```python
from build123d import *

# Parameters (mm, degrees)
SKETCH2_W           = 100
SKETCH2_H           = 200
BOSS_EXTRUDE1_DEPTH = 75
SKETCH5_R           = 2.5
SKETCH3_R           = 10
SKETCH6_R           = 2.5
CUT_EXTRUDE1_DEPTH  = 4


with BuildPart() as part:
    # Sketch2 → Boss-Extrude1 (new body)
    with BuildSketch(Plane(origin=(0, 0, 0), x_dir=(1, 0, 0), z_dir=(0, 1, 0))):
        Rectangle(SKETCH2_W, SKETCH2_H)
    extrude(amount=BOSS_EXTRUDE1_DEPTH)

    # Sketch5 → Loft1 section 0
    with BuildSketch(Plane.ZY.offset(55)):
        with Locations((0, 15)):
            Circle(SKETCH5_R)
    # Sketch3 → Loft1 section 1
    with BuildSketch(Plane.ZY.offset(50)):
        with Locations((0, 15)):
            Circle(SKETCH3_R)
    loft1 = loft()

    # Sketch6 → Cut-Extrude1 (cut)
    with BuildSketch(Plane.ZY.offset(55)):
        with Locations((0, 15)):
            Circle(SKETCH6_R)
    cut_extrude1 = extrude(amount=-CUT_EXTRUDE1_DEPTH, mode=Mode.SUBTRACT)

    # Mirror1: Loft1, Cut-Extrude1 across plane
    add(loft1.mirror(Plane(origin=(0, 0, 0), x_dir=(0, 0, 1), z_dir=(1, 0, 0))))
    add(cut_extrude1.mirror(Plane(origin=(0, 0, 0), x_dir=(0, 0, 1), z_dir=(1, 0, 0))), mode=Mode.SUBTRACT)


solid = part.part
```
Geometry check sheet. Reference: the model listing, model coordinates, mm. A direction names the side the tool comes from. Coordinates: 2 decimals unless noted, no trailing zeros. Write each loop counter-clockwise with the first axis right and the second up, starting at its lowest first coordinate (ties: lowest second). Pieces come first, ordered by that corner, then holes. Notation, with made-up numbers: M 9,48 L 26,48 A25 ccw 26,80 Z; hole C -18.75,32.25 d8. An arc over 180 degrees is marked long. Answer as a JSON object with one key per item and string values.
1. Section check B-B, the plane y = 56. Enter the section's corners in (x, z), plus the area to 3 significant figures.
Answers below:
{"outline": "M -50,-100 L 50,-100 L 50,100 L -50,100 Z", "area": "20,000 mm²"}
2. Tool access check on faces 5 (the cylindrical face through (53.03, 12.56, -0.54)), 6 (the flat face through (-1, 37, 100)), 7 (the flat face through (-51, 15, 0)). Record the directions out of +Z, -Z, +X, -X, +Y, -Y that give a thin tool (end or side, any length) a straight path to the whole face; none if there is none.
Answers below:
{"face 5": "+X", "face 6": "+Z, +X, -X, +Y, -Y", "face 7": "-X"}
3. Section check C-C, the plane z = 82.5. Enter the section's corners in (x, y), plus the area to 3 significant figures.
Answers below:
{"outline": "M -50,0 L 50,0 L 50,75 L -50,75 Z", "area": "7,500 mm²"}
4. Go/stop test with flat-tipped pins: pin 1 Ø4.5 at (y, z) = (15, 0) entering from +X; pin 2 Ø1.5 at (y, z) = (14.5, 1) entering from -X; pin 3 Ø5 at (y, z) = (8, 67) entering from +X. Record where each tip stops, or that it passes through.
Answers below:
{"pin 1": "stops at x = 51", "pin 2": "stops at x = -51", "pin 3": "stops at x = 50"}
5. Section check A-A, the plane z = 0. Enter the section's corners in (x, y), plus the area to 4 significant figures.
Answers below:
{"outline": "M -55,12.5 L -50,5 L -50,0 L 50,0 L 50,5 L 55,12.5 L 51,12.5 L 51,17.5 L 55,17.5 L 50,25 L 50,75 L -50,75 L -50,25 L -55,17.5 L -51,17.5 L -51,12.5 Z", "area": "7,585 mm²"}
6. Scan lines: L1, parallel to X at y = 23, z = 67.5; L2, parallel to Y at x = -53.45, z = 0 (3 decimals); L3, parallel to Y at x = -54, z = 0. Record each from-to range of solid material in increasing order.
Answers below:
{"L1": "x = -50 to 50", "L2": "y = 10.175 to 12.5, 17.5 to 19.825", "L3": "y = 11 to 12.5, 17.5 to 19"}
7. Draft check along Z on faces 1 (the flat face through (51, 15, 0)), 2 (the cylindrical face through (-53.03, 12.56, -0.54)), 3 (the conical face through (54.687, 12.101, -0.644)), 4 (the flat face through (50, 37, 1)). Enter one of: released by +Z, released by -Z, zero draft, split by the parting line, or undercut.
Answers below:
{"face 1": "undercut", "face 2": "undercut", "face 3": "split by the parting line", "face 4": "zero draft"}
